The model under review builds one solid part; all positions refer to its coordinate system, in mm. A direction names the side the tool comes from. Give positions to 0.01 mm unless a question says otherwise; leave off trailing zeros. Order: outer loops, then holes, each group sorted by start corner. A loop starts at its lowest first (then second) coordinate and runs counter-clockwise, first axis right, second up. Notation, with made-up numbers: (71.5, 33.5) -> (107.5, 33.5) arc R21 cw to (107.5, 59.5) -> close; hole circle Ø3 at (-26.5, 49.5). An arc over 180 degrees is marked (long way). Use one line per item in the form item = value.
```python
from build123d import *

# Parameters (mm, degrees)
SKETCH_1_W          = 255
SKETCH_1_H          = 80
EXTRUDE_1_DEPTH     = 5
SKETCH_2_R          = 5
CUT_EXTRUDE_1_DEPTH = 5
SKETCH_3_R          = 4
CUT_EXTRUDE_2_DEPTH = 10
SKETCH_4_W          = 88
SKETCH_4_H          = 20
EXTRUDE_2_DEPTH     = 10
SKETCH_5_R          = 15
CUT_EXTRUDE_3_DEPTH = 10
SKETCH_6_R          = 7
EXTRUDE_3_DEPTH     = 15
HOLE_WIZARD_M6_1_D  = 5
CUT_EXTRUDE_4_DEPTH = 7
HOLE_WIZARD_M4_1_D  = 3.3
FILLET_1_R          = 10
SKETCH_13_R         = 6.969385005
EXTRUDE_5_DEPTH     = 5
SKETCH_14_W         = 5
SKETCH_14_H         = 75
EXTRUDE_6_DEPTH     = 80
SKETCH_15_W         = 20
SKETCH_15_H         = 5
EXTRUDE_7_DEPTH     = 80
EXTRUDE_8_DEPTH     = 5
SKETCH_17_R         = 3
CUT_EXTRUDE_5_DEPTH = 5
FILLET_2_R          = 1
SKETCH_18_W         = 309.613912266
SKETCH_18_H         = 134.290371586
CUT_EXTRUDE_6_DEPTH = 81
SKETCH_19_R         = 17
CUT_EXTRUDE_7_DEPTH = 11
SKETCH_20_W         = 10
SKETCH_20_H         = 4.5
EXTRUDE_9_DEPTH     = 88
SKETCH_21_R         = 1.75
CUT_EXTRUDE_8_DEPTH = 11
SKETCH_22_R         = 3.25
CUT_EXTRUDE_9_DEPTH = 3.5
FILLET_4_R          = 1


with BuildPart() as part:
    # 草图1 → 凸台-拉伸1 (new body)
    with BuildSketch(Plane.XY):
        Rectangle(SKETCH_1_W, SKETCH_1_H)
    extrude(amount=EXTRUDE_1_DEPTH)

    # 草图2 → 切除-拉伸1 (cut)
    with BuildSketch(Plane.XY.offset(5)):
        with Locations((-107.5, 0)):
            Circle(SKETCH_2_R)
    extrude(amount=-CUT_EXTRUDE_1_DEPTH, mode=Mode.SUBTRACT)

    # 草图3 → 切除-拉伸2 (cut)
    with BuildSketch(Plane.XY.offset(5)):
        with Locations((-45, 0)):
            Circle(SKETCH_3_R)
    extrude(amount=-CUT_EXTRUDE_2_DEPTH, mode=Mode.SUBTRACT)

    # 草图4 → 凸台-拉伸2 (add)
    with BuildSketch(Plane.XY.offset(5)):
        with Locations((-9.5, 0)):
            Rectangle(SKETCH_4_W, SKETCH_4_H)
    extrude(amount=EXTRUDE_2_DEPTH)

    # 草图5 → 切除-拉伸3 (cut)
    with BuildSketch(Plane.XY.offset(5)):
        with Locations((70, 0)):
            Circle(SKETCH_5_R)
    extrude(amount=-CUT_EXTRUDE_3_DEPTH, mode=Mode.SUBTRACT)

    # 草图6 → 凸台-拉伸3 (add)
    with BuildSketch(Plane(origin=(0, 0, 0), x_dir=(-1, 0, 0), z_dir=(0, 0, -1))):
        with Locations((107.5, 0)):
            Circle(SKETCH_6_R)
    extrude(amount=-EXTRUDE_3_DEPTH)

    # M6 螺纹孔1 (through all)
    with Locations(Plane.XY.offset(15)):
        with Locations((-107.5, 0)):
            Hole(HOLE_WIZARD_M6_1_D / 2)

    # 草图10 → 切除-拉伸4 (cut)
    with BuildSketch(Plane.XY.offset(15)):
        with BuildLine():
            Line((-53.5, 5.1), (34.5, 5.1))
            ThreePointArc((34.5, 5.1), (39.6, 0), (34.5, -5.1))
            Line((34.5, -5.1), (-53.5, -5.1))
            ThreePointArc((-53.5, -5.1), (-58.6, 0), (-53.5, 5.1))
        make_face()
    extrude(amount=-CUT_EXTRUDE_4_DEPTH, mode=Mode.SUBTRACT)

    # M4 螺纹孔1 (through all)
    with Locations(Plane(origin=(0, 0, 0), x_dir=(-1, 0, 0), z_dir=(0, 0, -1))):
        with Locations((-39.75, -26.5), (-39.75, -1.5), (-109.94007449, -26.5), (-100.25, -1.5)):
            Hole(HOLE_WIZARD_M4_1_D / 2)

    # 圆角1
    fillet_1_edges = [part.edges().sort_by_distance(p)[0] for p in [
        (-127.5, 40, 2.5),
        (-127.5, -40, 2.5),
    ]]
    fillet(fillet_1_edges, radius=FILLET_1_R)

    # 草图13 → 凸台-拉伸5 (add)
    with BuildSketch(Plane.XY.offset(5)):
        with Locations((-45, 0)):
            Circle(SKETCH_13_R)
    extrude(amount=-EXTRUDE_5_DEPTH)

    # 草图14 → 凸台-拉伸6 (add)
    with BuildSketch(Plane.XZ.offset(40)):
        with Locations((125, -37.5)):
            Rectangle(SKETCH_14_W, SKETCH_14_H)
    extrude(amount=-EXTRUDE_6_DEPTH)

    # 草图15 → 凸台-拉伸7 (add)
    with BuildSketch(Plane.XZ.offset(40)):
        with Locations((112.5, -72.5)):
            Rectangle(SKETCH_15_W, SKETCH_15_H)
    extrude(amount=-EXTRUDE_7_DEPTH)

    # 草图16 → 凸台-拉伸8 (add)
    with BuildSketch(Plane.XZ.offset(40)):
        Polygon((-32.5, 5), (-32.5, 0), (102.5, -75), (127.5, -75), (127.5, 5), align=None)
    extrude_8 = extrude(amount=-EXTRUDE_8_DEPTH)

    # 镜向1: 凸台-拉伸8 across plane
    add(extrude_8.mirror(Plane.ZX))

    # 草图17 → 切除-拉伸5 (cut)
    with BuildSketch(Plane(origin=(0, 0, -75), x_dir=(-1, 0, 0), z_dir=(0, 0, -1))):
        with Locations((-114.5, -15)):
            Circle(SKETCH_17_R)
        with Locations((-114.5, 15)):
            Circle(SKETCH_17_R)
    extrude(amount=-CUT_EXTRUDE_5_DEPTH, mode=Mode.SUBTRACT)

    # 圆角2
    fillet_2_edges = [part.edges().sort_by_distance(p)[0] for p in [
        (-127.5, 0, 0),
        (-124.571067812, 37.071067812, 0),
        (-124.571067812, -37.071067812, 0),
        (-127.5, 0, 5),
        (-124.571067812, 37.071067812, 5),
        (-124.571067812, -37.071067812, 5),
        (127.5, 0, -75),
        (115, -40, -75),
        (115, 40, -75),
        (127.5, 0, 5),
        (35, -40, -37.5),
        (35, -35, -37.5),
        (5, 40, 5),
        (-75, 40, 0),
        (35, 40, -37.5),
        (35, 35, -37.5),
        (127.5, 40, -35),
        (127.5, -40, -35),
        (-75, -40, 0),
        (5, -40, 5),
    ]]
    fillet(fillet_2_edges, radius=FILLET_2_R)

    # 草图18 → 切除-拉伸6 (cut, through all)
    with BuildSketch(Plane.XY.offset(5)):
        Rectangle(SKETCH_18_W, SKETCH_18_H)
    extrude(amount=-CUT_EXTRUDE_6_DEPTH, mode=Mode.SUBTRACT)

    # 草图19 → 切除-拉伸7 (cut, through all)
    with BuildSketch(Plane.XY.offset(15)):
        with Locations((-107.5, 0)):
            Circle(SKETCH_19_R)
    extrude(amount=-CUT_EXTRUDE_7_DEPTH, mode=Mode.SUBTRACT)

    # 草图20 → 凸台-拉伸9 (add)
    with BuildSketch(Plane(origin=(34.5, 0, 0), x_dir=(0, 0, -1), z_dir=(1, 0, 0))):
        with Locations((-10, 12.25)):
            Rectangle(SKETCH_20_W, SKETCH_20_H)
    extrude_9 = extrude(amount=-EXTRUDE_9_DEPTH)

    # 镜向2: 凸台-拉伸9 across plane
    add(extrude_9.mirror(Plane.ZX))

    # 草图21 → 切除-拉伸8 (cut, through all)
    with BuildSketch(Plane.XY.offset(15)):
        with Locations((-42, 10)):
            Circle(SKETCH_21_R)
        with Locations((-9.5, 10)):
            Circle(SKETCH_21_R)
        with Locations((23, 10)):
            Circle(SKETCH_21_R)
        with Locations((23, -10)):
            Circle(SKETCH_21_R)
        with Locations((-9.5, -10)):
            Circle(SKETCH_21_R)
        with Locations((-42, -10)):
            Circle(SKETCH_21_R)
    extrude(amount=-CUT_EXTRUDE_8_DEPTH, mode=Mode.SUBTRACT)

    # 草图22 → 切除-拉伸9 (cut)
    with BuildSketch(Plane.XY.offset(15)):
        with Locations((-42, 10)):
            Circle(SKETCH_22_R)
        with Locations((-9.5, 10)):
            Circle(SKETCH_22_R)
        with Locations((23, 10)):
            Circle(SKETCH_22_R)
        with Locations((23, -10)):
            Circle(SKETCH_22_R)
        with Locations((-9.5, -10)):
            Circle(SKETCH_22_R)
        with Locations((-42, -10)):
            Circle(SKETCH_22_R)
    extrude(amount=-CUT_EXTRUDE_9_DEPTH, mode=Mode.SUBTRACT)

    # 圆角4
    fillet_4_edges = [part.edges().sort_by_distance(p)[0] for p in [
        (-9.5, 14.5, 15),
        (-9.5, -14.5, 15),
        (-9.5, 5.1, 15),
        (-9.5, -5.1, 15),
    ]]
    fillet(fillet_4_edges, radius=FILLET_4_R)


solid = part.part
```
1. For pin 1 Ø4 at (x, y) = (23, -10) entering from +Z, flat-tipped, find the tip position at first contact; note if it passes through.
Values:
pin_1 = 11.5
2. Add section D-D on z = 6.5. Give the boundary of the cut face in (x, y), then the cut area to 3 significant figures.
Values:
outline = (-53.5, -14.5) -> (34.5, -14.5) -> (34.5, 14.5) -> (-53.5, 14.5) -> close; hole circle Ø3.5 at (-42, -10); hole circle Ø3.5 at (-42, 10); hole circle Ø3.5 at (-9.5, -10); hole circle Ø3.5 at (-9.5, 10); hole circle Ø3.5 at (23, -10); hole circle Ø3.5 at (23, 10)
area = 2,490 mm^2
3. For L1, parallel to Y at x = -9.5, z = 13.8; L2, parallel to Y at x = -9.5, z = 7.75; L3, parallel to X at y = 9, z = 14, list the stretches that pass through material, from the lowest coordinate up.
Values:
L1 = -14.5 to -13.25, -6.75 to -5.1, 5.1 to 6.75, 13.25 to 14.5
L2 = -14.5 to -11.75, -8.25 to 8.25, 11.75 to 14.5
L3 = -53.5 to -45.09, -38.91 to -12.59, -6.41 to 19.91, 26.09 to 34.5
4. Add section C-C on x = -9.5. Give the boundary of the cut face in (y, z).
Values:
outline = (-14.5, 5) -> (-11.75, 5) -> (-11.75, 11.5) -> (-13.25, 11.5) -> (-13.25, 15) -> (-13.5, 15) arc R1 ccw to (-14.5, 14) -> close; (-8.25, 5) -> (8.25, 5) -> (8.25, 11.5) -> (6.75, 11.5) -> (6.75, 15) -> (6.1, 15) arc R1 ccw to (5.1, 14) -> (5.1, 8) -> (-5.1, 8) -> (-5.1, 14) arc R1 ccw to (-6.1, 15) -> (-6.75, 15) -> (-6.75, 11.5) -> (-8.25, 11.5) -> close; (11.75, 5) -> (14.5, 5) -> (14.5, 14) arc R1 ccw to (13.5, 15) -> (13.25, 15) -> (13.25, 11.5) -> (11.75, 11.5) -> close
5. Add section B-B on y = 10. Give the boundary of the cut face in (x, z), then the cut area to 4 significant figures.
Values:
outline = (-53.5, 5) -> (-43.75, 5) -> (-43.75, 11.5) -> (-45.25, 11.5) -> (-45.25, 15) -> (-53.5, 15) -> close; (-40.25, 5) -> (-11.25, 5) -> (-11.25, 11.5) -> (-12.75, 11.5) -> (-12.75, 15) -> (-38.75, 15) -> (-38.75, 11.5) -> (-40.25, 11.5) -> close; (-7.75, 5) -> (21.25, 5) -> (21.25, 11.5) -> (19.75, 11.5) -> (19.75, 15) -> (-6.25, 15) -> (-6.25, 11.5) -> (-7.75, 11.5) -> close; (24.75, 5) -> (34.5, 5) -> (34.5, 15) -> (26.25, 15) -> (26.25, 11.5) -> (24.75, 11.5) -> close
area = 743.5 mm^2
6. Add section A-A on z = 12.25. Give the boundary of the cut face in (x, y).
Values:
outline = (-53.5, -14.5) -> (34.5, -14.5) -> (34.5, -5.1) -> (-53.5, -5.1) -> close; (-53.5, 5.1) -> (34.5, 5.1) -> (34.5, 14.5) -> (-53.5, 14.5) -> close; hole circle Ø6.5 at (-42, -10); hole circle Ø6.5 at (-42, 10); hole circle Ø6.5 at (-9.5, -10); hole circle Ø6.5 at (-9.5, 10); hole circle Ø6.5 at (23, -10); hole circle Ø6.5 at (23, 10)
7. Tool access review of faces 3 (the face through (-9, 0, 8)), 4 (the face through (-8.6, -8.5, 8.3)), 5 (the face through (-40.6, 8.6, 11.5)): name each direction out of +Z, -Z, +X, -X, +Y, -Y from which nothing blocks a thin tool from reaching the whole face with its end or side.
Values:
face_3 = +Z, +X, -X
face_4 = +Z, -Z
face_5 = +Z
8. The part is to be moulded in two halves that separate along Y. For faces 1 (the face through (-8.9, -6.5, 15)), 2 (the face through (-11.895, 12.197, 13.274)), say which applies: +Y half, -Y half, draft (parallel to the pull), parting line (faces both ways), or undercut.
Values:
face_1 = draft
face_2 = undercut
